from build123d import *

# Parameters (mm, degrees)
SKETCH2_W           = 140
SKETCH2_H           = 100
BOSS_EXTRUDE1_DEPTH = 5
SKETCH3_W           = 100
SKETCH3_H           = 140
SKETCH3_W_2         = 90
SKETCH3_H_2         = 130
BOSS_EXTRUDE2_DEPTH = 30
BOSS_EXTRUDE3_START = 35
BOSS_EXTRUDE3_DEPTH = 50


with BuildPart() as part:
    # Sketch2 → Boss-Extrude1 (new body)
    with BuildSketch(Plane(origin=(0, 0, 0), x_dir=(0, 1, 0), z_dir=(0, 0, 1))):
        Rectangle(SKETCH2_W, SKETCH2_H)
    extrude(amount=BOSS_EXTRUDE1_DEPTH)

    # Sketch3 → Boss-Extrude2 (add)
    with BuildSketch(Plane.XY.offset(5)):
        Rectangle(SKETCH3_W, SKETCH3_H)
        Rectangle(SKETCH3_W_2, SKETCH3_H_2, mode=Mode.SUBTRACT)
    extrude(amount=BOSS_EXTRUDE2_DEPTH)

    # Sketch4 → Boss-Extrude3 (add)
    with BuildSketch(Plane(origin=(0, 0, 0), x_dir=(0, 1, 0), z_dir=(0, 0, 1)).offset(BOSS_EXTRUDE3_START)):
        Polygon((70, 50), (-70, 50), (-70, -50), (70, -50), (70, -45), (-65, -45), (-65, 45), (70, 45), align=None)
    extrude(amount=BOSS_EXTRUDE3_DEPTH)


solid = part.part
For this review, take the finished solid that the model builds, in its own axes (mm). A direction names the side the tool comes from. Give positions to 0.01 mm unless a question says otherwise; leave off trailing zeros. Loops run counter-clockwise (first coordinate to the right, second up) from the corner with the lowest first, then second, coordinate; pieces in that order, holes last.
Item 1: Take a section at B-B, the plane z = 38. State the section outline as (x, y) points, and give its area (3 significant figures).
Item 2: For line 1 along X through (y, z) = (5.5, 74); line 2 along Y through (x, z) = (8, 13); line 3 along Y through (x, z) = (-43, 41.5), list the stretches that pass through material, from the lowest coordinate up.
Item 3: Tool access review of faces 1 (the flat face through (-1, 68, 35)), 2 (the flat face through (45, 3, 44)), 3 (the flat face through (0, -68, 85)): name each direction out of +Z, -Z, +X, -X, +Y, -Y from which nothing blocks a thin tool from reaching the whole face with its end or side.
Item 4: Insertion check: pin 1 (6 mm diameter, centred on x = -10, y = -7.5, fed in from +Z); pin 2 (1 mm diameter, centred on x = -32, z = 39.5, fed in from +Y); pin 3 (1.5 mm diameter, centred on x = -7.5, y = 68, fed in from +Z). Each pin has a flat end and moves straight along its axis. Give the tip position at first contact, or say it passes through.
Item 5: Take a section at A-A, the plane x = 2. State the section outline as (y, z) points, and give its area (3 significant figures).
Item 6: Draft analysis for pull direction X (two halves, no side actions). For faces 4 (the flat face through (-1, 65, 20)), 5 (the flat face through (-1, -70, 42)), 6 (the flat face through (-50, 1, 42)), state which applies: +X half, -X half, draft (parallel to the pull), parting line (faces both ways), or undercut.
Item 7: Take a section at C-C, the plane z = 19. State the section outline as (x, y) points, and give its area (3 significant figures).
Calculated:
1. outline: (-50, -70) - (50, -70) - (50, 70) - (45, 70) - (45, -65) - (-45, -65) - (-45, 70) - (-50, 70) - close
1. area: 1,850 mm2
2. line 1: x = -50 to -45, 45 to 50
2. line 2: y = -70 to -65, 65 to 70
2. line 3: y = -70 to -65
3. face 1: +Z, +Y
3. face 2: +Z
3. face 3: +Z, +X, -X, +Y, -Y
4. pin 1: stops at z = 5
4. pin 2: stops at y = -65
4. pin 3: stops at z = 35
5. outline: (-70, 0) - (70, 0) - (70, 35) - (65, 35) - (65, 5) - (-65, 5) - (-65, 85) - (-70, 85) - close
5. area: 1,250 mm2
6. face 4: undercut
6. face 5: draft
6. face 6: -X half
7. outline: (-50, -70) - (50, -70) - (50, 70) - (-50, 70) - close; hole (-45, -65) - (45, -65) - (45, 65) - (-45, 65) - close
7. area: 2,300 mm2
